Part model, mm, in its own coordinate system. A direction names the side the tool comes from. Round coordinates to 2 decimals unless told otherwise and drop trailing zeros. Order: outer loops, then holes, each group sorted by start corner. A loop starts at its lowest first (then second) coordinate and runs counter-clockwise, first axis right, second up. Notation, with made-up numbers: (78, -5.5) - (82, -5.5) arc R16 ccw to (82, 25.5) - close; hole circle Ø5 at (27.5, 89). An arc over 180 degrees is marked (long way). Answer as a JSON object with one key per item and string values.
```python
from build123d import *

# Parameters (mm, degrees)
SKETCH_2_W               = 53.534
SKETCH_2_H               = 26.767
EXTRUDE_1_DEPTH          = 1000
EXTRUDE_2_DEPTH          = 5
SKETCH_8_W               = 53.534
SKETCH_8_H               = 26.767
CUT_EXTRUDE_2_DEPTH      = 1010
SKETCH_9_R               = 40
SKETCH_9_R_2             = 35
CUT_EXTRUDE_4_DEPTH      = 1010
SKETCH_10_R              = 3
CUT_EXTRUDE_7_DEPTH      = 1010
SKETCH_11_R              = 42
EXTRUDE_3_DEPTH          = 25.94125
SKETCH_9_2_R             = 40
SKETCH_9_2_R_2           = 35
CUT_EXTRUDE_8_DEPTH      = 23.94125
CUT_EXTRUDE_9_DEPTH      = 23.94125
CUT_EXTRUDE_9_DEPTH_BACK = 2000
SKETCH_8_2_W             = 53.534
SKETCH_8_2_H             = 26.767


with BuildPart() as part:
    # Sketch 2 → Extrude 1 (new body)
    with BuildSketch(Plane.XY):
        with BuildLine():
            Line((-26.767, 14.8835), (26.767, 14.8835))
            ThreePointArc((26.767, 14.8835), (27.827660172, 14.444160172), (28.267, 13.3835))
            Line((28.267, 13.3835), (28.267, -13.3835))
            ThreePointArc((28.267, -13.3835), (27.827660172, -14.444160172), (26.767, -14.8835))
            Line((26.767, -14.8835), (-26.767, -14.8835))
            ThreePointArc((-26.767, -14.8835), (-27.827660172, -14.444160172), (-28.267, -13.3835))
            Line((-28.267, -13.3835), (-28.267, 13.3835))
            ThreePointArc((-28.267, 13.3835), (-27.827660172, 14.444160172), (-26.767, 14.8835))
        make_face()
        Rectangle(SKETCH_2_W, SKETCH_2_H, mode=Mode.SUBTRACT)
    extrude(amount=EXTRUDE_1_DEPTH)

    # Sketch 6 → Extrude 2 (add)
    with BuildSketch(Plane(origin=(0, 0, 0), x_dir=(-1, 0, 0), z_dir=(0, 0, -1))):
        with BuildLine():
            Line((-19.929966526, 49.955317788), (19.929966526, 49.955317788))
            ThreePointArc((19.929966526, 49.955317788), (41.143169962, 41.168521224), (49.929966526, 19.955317788))
            Line((49.929966526, 19.955317788), (49.929966526, -19.955317788))
            ThreePointArc((49.929966526, -19.955317788), (41.143169962, -41.168521224), (19.929966526, -49.955317788))
            Line((19.929966526, -49.955317788), (-19.929966526, -49.955317788))
            ThreePointArc((-19.929966526, -49.955317788), (-41.143169962, -41.168521224), (-49.929966526, -19.955317788))
            Line((-49.929966526, -19.955317788), (-49.929966526, 19.955317788))
            ThreePointArc((-49.929966526, 19.955317788), (-41.143169962, 41.168521224), (-19.929966526, 49.955317788))
        make_face()
    extrude(amount=EXTRUDE_2_DEPTH)

    # Sketch 8 → Cut-Extrude 2 (cut)
    with BuildSketch(Plane.XY.offset(1000)):
        Rectangle(SKETCH_8_W, SKETCH_8_H)
    extrude(amount=-CUT_EXTRUDE_2_DEPTH, mode=Mode.SUBTRACT)

    # Sketch 9 → Cut-Extrude 4 (cut)
    with BuildSketch(Plane(origin=(0, 0, -5), x_dir=(-1, 0, 0), z_dir=(0, 0, -1))):
        Circle(SKETCH_9_R)
        Circle(SKETCH_9_R_2, mode=Mode.SUBTRACT)
    extrude(amount=-CUT_EXTRUDE_4_DEPTH, mode=Mode.SUBTRACT)


with BuildPart() as cut_extrude_4_piece_1:
    # of the separate pieces the step leaves, piece 1, a body of its own (cut_extrude_4_pieces)
    add(part.part.solids().sort_by_distance((-35, 0, 0))[0])



with BuildPart() as cut_extrude_4_piece_2:
    # of the separate pieces the step leaves, piece 2, a body of its own (cut_extrude_4_pieces)
    add(part.part.solids().sort_by_distance((19.929966526, 49.955317788, 0))[0])

    # Sketch 10 → Cut-Extrude 7 (cut)
    with BuildSketch(Plane(origin=(0, 0, -5), x_dir=(-1, 0, 0), z_dir=(0, 0, -1))):
        with Locations((-35, 35)):
            Circle(SKETCH_10_R)
        with Locations((-35, -35)):
            Circle(SKETCH_10_R)
        with Locations((35, -35)):
            Circle(SKETCH_10_R)
        with Locations((35, 35)):
            Circle(SKETCH_10_R)
    extrude(amount=-CUT_EXTRUDE_7_DEPTH, mode=Mode.SUBTRACT)


with BuildPart() as cut_extrude_4_piece_1_1:
    add(cut_extrude_4_piece_1.part)

    add(cut_extrude_4_piece_2.part)  # Extrude 3 merges Cut-Extrude 4 piece 2
    # Sketch 11 → Extrude 3 (add)
    with BuildSketch(Plane(origin=(0, 0, -5), x_dir=(-1, 0, 0), z_dir=(0, 0, -1))):
        Circle(SKETCH_11_R)
    extrude(amount=-EXTRUDE_3_DEPTH)

    # Sketch 9_2 → Cut-Extrude 8 (cut)
    with BuildSketch(Plane(origin=(0, 0, -5), x_dir=(-1, 0, 0), z_dir=(0, 0, -1))):
        Circle(SKETCH_9_2_R)
        Circle(SKETCH_9_2_R_2, mode=Mode.SUBTRACT)
    extrude(amount=-CUT_EXTRUDE_8_DEPTH, mode=Mode.SUBTRACT)

    # Sketch 8_2 → Cut-Extrude 9 (cut, two sides: drawn at the far end of the back side and taken through both)
    with BuildSketch(Plane.XY.offset(1000).offset(-CUT_EXTRUDE_9_DEPTH_BACK)):
        Rectangle(SKETCH_8_2_W, SKETCH_8_2_H)
    extrude(amount=CUT_EXTRUDE_9_DEPTH + CUT_EXTRUDE_9_DEPTH_BACK, mode=Mode.SUBTRACT)


solid = cut_extrude_4_piece_1_1.part
```
Item 1: Probe L1, parallel to Y at x = -21, z = 566; L2, parallel to X at y = 11, z = 942; L3, parallel to Z at x = -16.5, y = -34.5. List the from-to ranges inside material, lowest first. Write a range as from..to.
Taken from the geometry:
{"L1": "-14.88..-13.38, 13.38..14.88", "L2": "-28.27..-26.77, 26.77..28.27", "L3": "18.94..20.94"}
Item 2: Tool access for faces 1 (the flat face through (-28.267, 0, 504)), 2 (the flat face through (28.267, 0, 504)), 3 (the cylindrical face through (8.67, -39.05, 6.8)): list every direction of +Z, -Z, +X, -X, +Y, -Y with a clear straight run to the whole face (end or side of a thin tool).
Taken from the geometry:
{"face 1": "+Z, -X, +Y, -Y", "face 2": "+Z, +X, +Y, -Y", "face 3": "-Z"}
Item 3: Two-plate mould, pull along X, no slides. Class faces 4 (the flat face through (0, -13.384, 490)), 5 (the cylindrical face through (-40.06, 12.62, 10.32)), 6 (the flat face through (0, -14.884, 504)): pulls with the +X half, pulls with the -X half, needs draft (parallel to the pull), parting line crosses it, or undercut.
Taken from the geometry:
{"face 4": "undercut", "face 5": "parting line crosses it", "face 6": "needs draft"}
Item 4: Drop flat-ended pins along their axis: P1, Ø12, axis at y = -12, z = 238.5, coming from the +X side; P2, Ø8, axis at y = 5.5, z = 271.5, coming from the -X side; P3, Ø8, axis at x = 8, z = 132.5, coming from the -Y side. Give the stop position or say it passes through.
Taken from the geometry:
{"P1": "x = 28.27", "P2": "x = -28.27", "P3": "y = -14.88"}
Item 5: Cut at B-B (z = 124.5). Write the cut outline in (x, y), plus the area to 3 significant figures.
Taken from the geometry:
{"outline": "(-28.27, -13.38) arc R1.5 ccw to (-26.77, -14.88) - (26.77, -14.88) arc R1.5 ccw to (28.27, -13.38) - (28.27, 13.38) arc R1.5 ccw to (26.77, 14.88) - (-26.77, 14.88) arc R1.5 ccw to (-28.27, 13.38) - close; hole (-26.77, -13.38) - (26.77, -13.38) - (26.77, 13.38) - (-26.77, 13.38) - close", "area": "248 mm2"}
Item 6: Cut at A-A (x = 0). Write the cut outline in (y, z), plus the area to 3 significant figures.
Taken from the geometry:
{"outline": "(-49.96, -5) - (-40, -5) - (-40, 18.94) - (-35, 18.94) - (-35, -5) - (-13.38, -5) - (-13.38, 1000) - (-14.88, 1000) - (-14.88, 20.94) - (-42, 20.94) - (-42, 0) - (-49.96, 0) - close; (13.38, -5) - (35, -5) - (35, 18.94) - (40, 18.94) - (40, -5) - (49.96, -5) - (49.96, 0) - (42, 0) - (42, 20.94) - (14.88, 20.94) - (14.88, 1000) - (13.38, 1000) - close", "area": "4,260 mm2"}
